Work out the finished part from the listing and answer in its coordinate system (mm). Face numbers are marked on the shaded views. Give positions to 0.01 mm unless a question says otherwise; leave off trailing zeros. Order: outer loops, then holes, each group sorted by start corner. A loop starts at its lowest first (then second) coordinate and runs counter-clockwise, first axis right, second up. Notation, with made-up numbers: (19, -27) -> (39, -27) arc R27 ccw to (39, 1) -> close; hole circle Ø11 at (37.25, -20). An arc over 180 degrees is marked (long way). Answer as CSV lines item,"result". Start each with the question number.
1. Find the intervals of material crossed by L1, parallel to X at y = -7.5, z = 190; L2, parallel to Z at x = 5, y = -12.5; L3, parallel to Z at x = 0.5, y = -12, in increasing order.
2. For a pull along Z with two mould halves and no side action, classify the marked faces 1, 2 and 3 as released by +Z, released by -Z, zero draft, split by the parting line, or undercut.
3. A flat-ended cylindrical pin translates along its axis: pin 1 (1.5 mm diameter, centred on x = 14.5, y = -11, fed in from +Z). Find the tip coordinate at first contact, or state that the pin passes through.
4. A cutting plane is placed at A-A (x = 17). Give the vertices of the cut face in (y, z), then the cut area to 3 significant figures.
from build123d import *

# Parameters (mm, degrees)
F0_W     = 88.9
F0_H     = 457.2
F1_DEPTH = 44.45
F3_DEPTH = 127
F4_R     = 6.35
F5_DEPTH = 127


with BuildPart() as f1:
    # F0 (on Front) → F1 (new body, symmetric)
    with BuildSketch(Plane.XZ):
        Rectangle(F0_W, F0_H)
    extrude(amount=F1_DEPTH, both=True)

    # F2 (on Right) → F3 (cut, symmetric)
    with BuildSketch(Plane.YZ):
        Polygon((44.45, 177.8), (44.45, 228.6), (36.1311809715, 228.6), align=None)
        Polygon((-42.3455583973, 215.7489410875), (36.1311809715, 228.6), (34.0267393688, 241.4510589125), (-44.45, 228.6), align=None)
        Polygon((-32.2976503157, 154.3900235786), (-42.3455583973, 215.7489410875), (-44.45, 228.6), (-44.45, 152.4), align=None)
    extrude(amount=F3_DEPTH, both=True, mode=Mode.SUBTRACT)

    # F4 (on face) → F5 (cut, symmetric)
    with BuildSketch(Plane(origin=(0, -6.8321038597, -1.1187999132), x_dir=(1, 0, 0), z_dir=(0, -0.9868557164, -0.1616038211))):
        with Locations((0, 194.3562798646)):
            Circle(F4_R)
    extrude(amount=F5_DEPTH, both=True, mode=Mode.SUBTRACT)


solid = f1.part
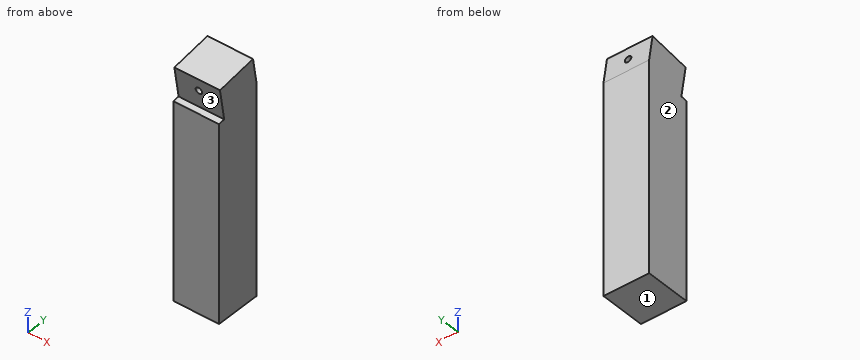
Answer sheet:
1,L1,"x = -44.45 to -2.91, 2.91 to 44.45"
1,L2,"z = -228.6 to 190.93, 198.86 to 220.64"
1,L3,"z = -228.6 to 188.57, 201.39 to 220.72"
2,face 1,"released by -Z"
2,face 2,"zero draft"
2,face 3,"undercut"
3,pin 1,"stops at z = 221"
4,outline,"(-44.45, -228.6) -> (44.45, -228.6) -> (44.45, 177.8) -> (36.13, 228.6) -> (-42.35, 215.75) -> (-32.3, 154.39) -> (-44.45, 152.4) -> close"
4,area,"39,500 mm^2"
